Source: CAD feature listing. Evaluate the final solid. Frame: model axes, mm. Round coordinates to 2 decimals unless told otherwise and drop trailing zeros. Write each loop counter-clockwise with the first axis right and the second up, starting at its lowest first coordinate (ties: lowest second). Pieces come first, ordered by that corner, then holes.
from build123d import *

# Parameters (mm, degrees)
SKETCH1_W                       = 250
SKETCH1_H                       = 250
BOSS_EXTRUDE1_DEPTH             = 1.25
SKETCH2_W                       = 240
SKETCH2_H                       = 240
CUT_EXTRUDE1_DEPTH              = 1
SKETCH3_R                       = 2.5
BOSS_EXTRUDE2_DEPTH             = 1
FILLET1_R                       = 2
TAP_DRILL_FOR_M3X0_5_TAP1_D     = 2.5
TAP_DRILL_FOR_M3X0_5_TAP1_DEPTH = 1.5
TAP_DRILL_FOR_M3X0_5_TAP1_TIP   = 0.751075774


with BuildPart() as part:
    # Sketch1 → Boss-Extrude1 (new, symmetric)
    with BuildSketch(Plane(origin=(0, 0, 0), x_dir=(1, 0, 0), z_dir=(0, 1, 0))):
        Rectangle(SKETCH1_W, SKETCH1_H)
    extrude(amount=BOSS_EXTRUDE1_DEPTH, both=True)

    # Sketch2 → Cut-Extrude1 (cut)
    with BuildSketch(Plane(origin=(0, 1.25, 0), x_dir=(1, 0, 0), z_dir=(0, 1, 0))):
        Rectangle(SKETCH2_W, SKETCH2_H)
    extrude(amount=-CUT_EXTRUDE1_DEPTH, mode=Mode.SUBTRACT)

    # Sketch3 → Boss-Extrude2 (add)
    with BuildSketch(Plane(origin=(0, 0.25, 0), x_dir=(1, 0, 0), z_dir=(0, 1, 0))):
        with Locations(Location((-115, -115, 0), (0, 0, 90))):
            Circle(SKETCH3_R)
        with Locations(Location((-85, -115, 0), (0, 0, 90))):
            Circle(SKETCH3_R)
        with Locations(Location((-55, -105, 0), (0, 0, 90))):
            Circle(SKETCH3_R)
        with Locations(Location((-15, -115, 0), (0, 0, 90))):
            Circle(SKETCH3_R)
        with Locations(Location((15, -115, 0), (0, 0, 90))):
            Circle(SKETCH3_R)
        with Locations(Location((55, -105, 0), (0, 0, 90))):
            Circle(SKETCH3_R)
        with Locations(Location((85, -115, 0), (0, 0, 90))):
            Circle(SKETCH3_R)
        with Locations(Location((-115, 115, 0), (0, 0, 90))):
            Circle(SKETCH3_R)
        with Locations(Location((-115, 85, 0), (0, 0, 90))):
            Circle(SKETCH3_R)
        with Locations(Location((-105, 55, 0), (0, 0, 90))):
            Circle(SKETCH3_R)
        with Locations(Location((-115, 15, 0), (0, 0, 90))):
            Circle(SKETCH3_R)
        with Locations(Location((-115, -15, 0), (0, 0, 90))):
            Circle(SKETCH3_R)
        with Locations(Location((-105, -55, 0), (0, 0, 90))):
            Circle(SKETCH3_R)
        with Locations(Location((-115, -85, 0), (0, 0, 90))):
            Circle(SKETCH3_R)
        with Locations(Location((115, 115, 0), (0, 0, 90))):
            Circle(SKETCH3_R)
        with Locations(Location((85, 115, 0), (0, 0, 90))):
            Circle(SKETCH3_R)
        with Locations(Location((55, 105, 0), (0, 0, 90))):
            Circle(SKETCH3_R)
        with Locations(Location((15, 115, 0), (0, 0, 90))):
            Circle(SKETCH3_R)
        with Locations(Location((-15, 115, 0), (0, 0, 90))):
            Circle(SKETCH3_R)
        with Locations(Location((-55, 105, 0), (0, 0, 90))):
            Circle(SKETCH3_R)
        with Locations(Location((-85, 115, 0), (0, 0, 90))):
            Circle(SKETCH3_R)
        with Locations(Location((115, -115, 0), (0, 0, 90))):
            Circle(SKETCH3_R)
        with Locations(Location((115, -85, 0), (0, 0, 90))):
            Circle(SKETCH3_R)
        with Locations(Location((105, -55, 0), (0, 0, 90))):
            Circle(SKETCH3_R)
        with Locations(Location((115, -15, 0), (0, 0, 90))):
            Circle(SKETCH3_R)
        with Locations(Location((115, 15, 0), (0, 0, 90))):
            Circle(SKETCH3_R)
        with Locations(Location((105, 55, 0), (0, 0, 90))):
            Circle(SKETCH3_R)
        with Locations(Location((115, 85, 0), (0, 0, 90))):
            Circle(SKETCH3_R)
        with Locations(Location((-35, 35, 0), (0, 0, 90))):
            Circle(SKETCH3_R)
        with Locations(Location((-35, -35, 0), (0, 0, 90))):
            Circle(SKETCH3_R)
        with Locations(Location((35, -35, 0), (0, 0, 90))):
            Circle(SKETCH3_R)
        with Locations(Location((35, 35, 0), (0, 0, 90))):
            Circle(SKETCH3_R)
    extrude(amount=BOSS_EXTRUDE2_DEPTH)

    # Fillet1
    fillet1_edges = [part.edges().sort_by_distance(p)[0] for p in [
        (120, 0.75, -120),
        (120, 0.75, 120),
        (-120, 0.75, 120),
        (-120, 0.75, -120),
        (125, 0, 125),
        (-125, 0, 125),
        (-125, 0, -125),
        (125, 0, -125),
    ]]
    fillet(fillet1_edges, radius=FILLET1_R)

    # Tap Drill for M3x0.5 Tap1
    with Locations(Plane(origin=(-115, 1.25, 115), x_dir=(0, 0, 1), z_dir=(0, 1, 0))):
        with Locations((0, 0), (0, 30), (-30, 0), (-60, 10), (-100, 0), (-130, 0), (-200, 0), (-170, 10), (-230, 0), (-230, 30), (-220, 60), (-230, 100), (-230, 130), (-150, 80), (-150, 150), (-10, 60), (-80, 80), (-80, 150), (0, 100), (0, 130), (-10, 170), (0, 200), (0, 230), (-30, 230), (-60, 220), (-100, 230), (-130, 230), (-170, 220), (-220, 170), (-230, 200), (-230, 230), (-200, 230)):
            Hole(TAP_DRILL_FOR_M3X0_5_TAP1_D / 2, depth=TAP_DRILL_FOR_M3X0_5_TAP1_DEPTH)
            with Locations((0, 0, -(TAP_DRILL_FOR_M3X0_5_TAP1_DEPTH + TAP_DRILL_FOR_M3X0_5_TAP1_TIP / 2))):  # 118° drill point
                Cone(0, TAP_DRILL_FOR_M3X0_5_TAP1_D / 2, TAP_DRILL_FOR_M3X0_5_TAP1_TIP, mode=Mode.SUBTRACT)


solid = part.part
1) Contact query for flat-ended pins moving along their axis: P1, Ø1.5, axis at x = -115, z = 115, coming from the +Y side; P2, Ø2, axis at x = 105, z = 55, coming from the +Y side; P3, Ø10, axis at x = -61.5, z = 85, coming from the +Y side. Output: stop coordinate, or through.
Taken from the geometry:
P1: stops at y = -0.55
P2: stops at y = -0.4
P3: stops at y = 0.25
2) Section query A-A on x = -49.5. Return the cut outline in (y, z), then the cut area to 3 significant figures.
Taken from the geometry:
outline: (-1.25, -125) - (1.25, -125) - (1.25, -120) - (0.25, -120) - (0.25, 120) - (1.25, 120) - (1.25, 125) - (-1.25, 125) - close
area: 385 mm2
3) Pull-direction query (Z, two-part tool) for faces 1 (the face through (-2, 0.25, -2)), 2 (the face through (-121, 1.25, -56)); classes: released by +Z, released by -Z, zero draft, split by the parting line, or undercut.
Taken from the geometry:
face 1: undercut
face 2: zero draft
4) Material intervals for line 1 (X direction, y = 0.5, z = 15); line 2 (X direction, y = 0.2, z = 15), sorted ascending.
Taken from the geometry:
line 1: x = -125 to -120, -117.5 to -116.25, -113.75 to -112.5, 112.5 to 113.75, 116.25 to 117.5, 120 to 125
line 2: x = -125 to -116.25, -113.75 to 113.75, 116.25 to 125
